Can you work these out from the model? Positions are in its coordinate system, mm. A direction names the side the tool comes from. Round coordinates to 2 decimals unless told otherwise and drop trailing zeros. Write each loop counter-clockwise with the first axis right and the second up, starting at its lowest first coordinate (ties: lowest second). Pieces come first, ordered by that corner, then holes.
Q1. If we section it at B-B (x = -18.5): Please give me the cut outline in (y, z).
Q2. For faces 4 (the flat face through (-9, -302, 10)), 5 (the flat face through (-9, -271, 0)), 6 (the flat face through (-9, -136, 2100)), 7 (the flat face through (-665, -30, 1065)), which set-ups out of +Z, -Z, +X, -X, +Y, -Y let a thin tool reach every point of the face, with its end or its side?
Q3. Please list where these lines run through material, in increasing order: line 1 along X through (y, z) = (-37.5, 976); line 2 along Z through (x, y) = (-421, -111.5); line 3 along Y through (x, z) = (436.5, 1059.5).
Q4. If we section it at A-A (y = -435.5): Please give me the cut outline in (x, z), plus the area to 3 significant figures.
Q5. I'm going to push flat-ended pins straight in: pin 1 Ø4 at (x, z) = (330, 250) entering from +Y; pin 2 Ø4 at (x, z) = (80.5, 1682.5) entering from -Y; pin 3 Ø8 at (x, z) = (669.5, 1352) entering from -Y. Where does each tip first touch, or does it pass through?
Q6. We'd pull the mould along Y, two halves only. Please class faces 1 (the flat face through (-675, -218, 1070)), 2 (the flat face through (669.93, -377.45, 1286.27)), 3 (the flat face through (-9, -540, 61)): +Y half, -Y half, draft (parallel to the pull), parting line (faces both ways), or undercut.
Q7. If we section it at C-C (z = 540): Please give me the cut outline in (x, y), plus the area to 3 significant figures.
Autodesk Inventor part; units mm, degrees
ref_plane "YZ Plane" through (0, 0, 0) normal (1, 0, 0) x (0, 1, 0)
ref_plane "XZ Plane" through (0, 0, 0) normal (0, 1, 0) x (-1, 0, 0)
ref_plane "XY Plane" through (0, 0, 0) normal (0, 0, 1) x (1, 0, 0)
sketch "Sketch1" plane through (0, 0, 0) normal (1, 0, 0) x (0, 1, 0)
  line L0 (0, 0) -> (-550, 0)
  line L1 (0, 0) -> (0, 2110)
  line L2 (-550, 0) -> (-550, 495)
  line L3 (-550, 495) -> (-200, 2100)
  line L4 (0, 2110) -> (-200, 2110)
  line L5 (-200, 2110) -> (-200, 2100)
  line L6 (-475, 395) -> (-145, 395)
  line L7 (-120, 370) -> (-120, 135)
  line L8 (-145, 110) -> (-475, 110)
  line L9 (-500, 135) -> (-500, 370)
  arc A0 (-475, 395) -> (-500, 370) centre (-475, 370) ccw
  arc A1 (-500, 135) -> (-475, 110) centre (-475, 135) ccw
  arc A2 (-145, 110) -> (-120, 135) centre (-145, 135) ccw
  arc A3 (-120, 370) -> (-145, 395) centre (-145, 370) ccw
  line L10 (-110, 1420) -> (-110, 1420)
  line L11 (-85, 1395) -> (-85, 1295)
  line L12 (-110, 1270) -> (-110, 1270)
  line L13 (-135, 1295) -> (-135, 1395)
  arc A4 (-110, 1420) -> (-135, 1395) centre (-110, 1395) ccw
  arc A5 (-85, 1395) -> (-110, 1420) centre (-110, 1395) ccw
  arc A6 (-110, 1270) -> (-85, 1295) centre (-110, 1295) ccw
  arc A7 (-135, 1295) -> (-110, 1270) centre (-110, 1295) ccw
  point P0 (-120, 110)
  point P1 (-500, 110)
  point P2 (-85, 1270)
  point P3 (-85, 1420)
  point P4 (-135, 1270)
  dimension "d0" = 550
  dimension "d1" = 2110
  dimension "d2" = 495
  dimension "d3" = 200
  dimension "d4" = 10
  dimension "d5" = 380
  dimension "d6" = 285
  dimension "d10" = 110
  dimension "d11" = 120
  dimension "d12" = 25
  dimension "d13" = 50
  dimension "d14" = 150
  dimension "d15" = 1270
  dimension "d16" = 85
  dimension "d17" = 25
extrude "Extrusion1" add sketch "Sketch1" along normal mid plane 1350
sketch "Sketch2" plane through (-675, 0, 2110) normal (0, 1, 0) x (1, 0, 0)
  line L0 (1340, 10) -> (10, 10)
  line L1 (10, 10) -> (10, 2110)
  line L2 (10, 2110) -> (1340, 2110)
  line L3 (1340, 2110) -> (1340, 10)
  line L4 (0, 0) -> (1350, 0)
  line L5 (1350, 2110) -> (1350, 0)
  line L6 (0, 0) -> (0, 2110)
  line L7 (0, 2110) -> (1350, 2110)
  point P0 (675, 2110)
  dimension "d20" = 10
  dimension "d21" = 10
  dimension "d22" = 10
  dimension "d23" = 0
extrude "Extrusion2" cut sketch "Sketch2" against normal blind 60 contours L0 L1 L2 L3
sketch "Sketch3" plane through (-675, -550, 0) normal (0, -1, 0) x (1, 0, 0)
  line L0 (10, 2100) -> (1340, 2100)
  line L1 (1340, 2100) -> (1340, 110)
  line L2 (1340, 110) -> (10, 110)
  line L3 (10, 110) -> (10, 2100)
  line L4 (1350, 2100) -> (1350, 495)
  line L5 (0, 495) -> (0, 2100)
  line L6 (1350, 2110) -> (0, 2110)
  line L7 (0, 0) -> (1350, 0)
  point P0 (675, 0)
  dimension "d26" = 10
  dimension "d27" = 10
  dimension "d28" = 10
  dimension "d29" = 110
extrude "Extrusion3" cut sketch "Sketch3" against normal blind 480
sketch "Sketch4" plane through (675, -475, 110) normal (0, 0, 1) x (1, 0, 0)
  line L0 (-1340, -65) -> (-10, -65)
  line L1 (-10, -65) -> (-10, 405)
  line L2 (-10, 405) -> (-1340, 405)
  line L3 (-1340, 405) -> (-1340, -65)
  line L4 (-1350, -75) -> (-1350, 275)
  line L5 (-10, -75) -> (-1340, -75)
  line L6 (0, 275) -> (0, -75)
  line L7 (-1340, 415) -> (-10, 415)
  point P0 (-675, 475)
  dimension "d32" = 10
  dimension "d33" = 10
  dimension "d34" = 10
  dimension "d35" = 10
extrude "Extrusion4" cut sketch "Sketch4" against normal blind 100
properties part number "Стенд"
A:
1. outline: (-550, 0) - (-60, 0) - (-60, 2100) - (0, 2100) - (0, 2110) - (-200, 2110) - (-200, 2100) - (-70, 2100) - (-70, 10) - (-540, 10) - (-540, 110) - (-550, 110) - close
2. face 4: none
2. face 5: -Z, +X, -X, +Y, -Y
2. face 6: -Y
2. face 7: -Z, +Y
3. line 1: x = -675 to -665, 665 to 675
3. line 2: z = 0 to 10, 2100 to 2110
3. line 3: y = -70 to -60
4. outline: (-675, 0) - (675, 0) - (675, 110) - (665, 110) - (665, 10) - (-665, 10) - (-665, 110) - (-675, 110) - close; (-675, 395) - (-665, 395) - (-665, 1020.06) - (-675, 1020.06) - close; (665, 395) - (675, 395) - (675, 1020.06) - (665, 1020.06) - close
4. area: 28,000 mm2
5. pin 1: stops at y = -60
5. pin 2: stops at y = -70
5. pin 3: stops at y = -363.99
6. face 1: draft
6. face 2: -Y half
6. face 3: undercut
7. outline: (-675, -540.19) - (-665, -540.19) - (-665, -70) - (665, -70) - (665, -540.19) - (675, -540.19) - (675, 0) - (665, 0) - (665, -60) - (-665, -60) - (-665, 0) - (-675, 0) - close
7. area: 24,100 mm2
